Work out the finished part from the listing and answer in its coordinate system (mm). A direction names the side the tool comes from. Round coordinates to 2 decimals unless told otherwise and drop trailing zeros. Return JSON: item names as keys, results as strings.
from build123d import *

# Parameters (mm, degrees)
SKETCH1_R           = 1.5
SKETCH1_W           = 31.5
SKETCH1_H           = 21.75
BOSS_EXTRUDE2_DEPTH = 12.9
SKETCH4_W           = 31.5
SKETCH4_H           = 21.75
BOSS_EXTRUDE3_DEPTH = 8.6


with BuildPart() as part:
    # Sketch1 → Boss-Extrude2 (new body)
    with BuildSketch(Plane.XY):
        with BuildLine():
            Line((-27.5, -17), (-27.5, 17))
            add(Edge.make_bspline(
                [(-27.5, 17), (-7.117727258, 20.399822972), (10.514459211, 15.859666911), (27.5, 0)],
                knots=[0, 0, 0, 0, 1, 1, 1, 1], degree=3))
            add(Edge.make_bspline(
                [(-27.5, -17), (-7.117727258, -20.399822972), (10.514459211, -15.859666911), (27.5, 0)],
                knots=[0, 0, 0, 0, 1, 1, 1, 1], degree=3))
        make_face()
        with Locations(Location((-25, 13, 0), (0, 0, 180))):
            Circle(SKETCH1_R, mode=Mode.SUBTRACT)
        with Locations(Location((-12.5, 16, 0), (0, 0, 180))):
            Circle(SKETCH1_R, mode=Mode.SUBTRACT)
        with Locations(Location((21.5, 0, 0), (0, 0, 180))):
            Circle(SKETCH1_R, mode=Mode.SUBTRACT)
        with Locations(Location((13.5, 0, 0), (0, 0, 180))):
            Circle(SKETCH1_R, mode=Mode.SUBTRACT)
        with Locations(Location((-12.5, -16, 0), (0, 0, 180))):
            Circle(SKETCH1_R, mode=Mode.SUBTRACT)
        with Locations(Location((-25, -13, 0), (0, 0, 180))):
            Circle(SKETCH1_R, mode=Mode.SUBTRACT)
        with Locations((-6.95, 0)):
            Rectangle(SKETCH1_W, SKETCH1_H, mode=Mode.SUBTRACT)
    extrude(amount=BOSS_EXTRUDE2_DEPTH)

    # Sketch4 → Boss-Extrude3 (add)
    with BuildSketch(Plane(origin=(0, 0, 0), x_dir=(-1, 0, 0), z_dir=(0, 0, -1))):
        with Locations((6.95, 0)):
            Rectangle(SKETCH4_W, SKETCH4_H)
    extrude(amount=-BOSS_EXTRUDE3_DEPTH)


solid = part.part
1) A tool of negligible diameter and unlimited length cuts with its end or side. For faces 3 (the cylindrical face through (15, 0, 6)), 4 (the flat face through (-22.7, 0, 11)), from which of +Z, -Z, +X, -X, +Y, -Y can it reach the whole face along a straight path? Write none if from no direction.
Verdict:
{"face 3": "+Z, -Z", "face 4": "+Z"}
2) Section A-A (z = 2.5) is taken. Count the separate pieces of the cut face and the enclosed holes in it, and give its area (3 significant figures).
Verdict:
{"separate pieces": "1", "enclosed holes": "6", "area": "1,450 mm2"}
3) Find the intervals of material crossed by L1, parallel to X at y = -0.5, z = 5.25; L2, parallel to Y at x = -12, z = 5.5; L3, parallel to Y at x = -25, z = 7, in increasing order.
Verdict:
{"L1": "x = -27.5 to 12.09, 14.91 to 20.09, 22.91 to 26.96", "L2": "y = -17.98 to -17.41, -14.59 to 14.59, 17.41 to 17.98", "L3": "y = -17.38 to -14.5, -11.5 to 11.5, 14.5 to 17.38"}
4) Determine the mould class of faces 1 (the flat face through (8.8, 0, 11)), 2 (the flat face through (-2, 12, 12.9)) for opening direction Y: pulls with the +Y half, pulls with the -Y half, needs draft (parallel to the pull), parting line crosses it, or undercut.
Verdict:
{"face 1": "undercut", "face 2": "needs draft"}
5) Flat-ended cylindrical pins translate along their axes: pin 1 (5 mm diameter, centred on x = -18.5, z = 1.5, fed in from -Y); pin 2 (1.5 mm diameter, centred on y = 9.5, z = 7.5, fed in from +X); pin 3 (2.5 mm diameter, centred on x = -25, y = 13, fed in from +Z); pin 4 (4 mm diameter, centred on y = 9.5, z = 5, fed in from +X). Find the tip coordinate at first contact, or state that the pin passes through.
Verdict:
{"pin 1": "stops at y = -18.06", "pin 2": "stops at x = 16.35", "pin 3": "passes through", "pin 4": "stops at x = 18.23"}
